Can you work these out from the model? Positions are in its coordinate system, mm. A direction names the side the tool comes from. Give positions to 0.01 mm unless a question says otherwise; leave off trailing zeros. Order: outer loops, then holes, each group sorted by start corner. A loop starts at its lowest first (then second) coordinate and runs counter-clockwise, first axis right, second up. Notation, with made-up numbers: M -5.75,36 L 28.25,36 A8 cw 28.25,40 Z; hole C 26,11.5 d7. An arc over 180 degrees is marked long. One line per question, with ' | ' between items. Start each with the question number.
1) For faces 4 (the flat face through (24, 1, 3.175)), 5 (the flat face through (26.035, 1, -2)), 6 (the flat face through (-26.035, 1, -2)), 7 (the flat face through (-9.525, 8, -5)), which set-ups out of +Z, -Z, +X, -X, +Y, -Y let a thin tool reach every point of the face, with its end or its side?
2) If we section it at C-C, the plane z = 2.25: Please give me the cut outline in (x, y) (3 decimals), plus the area to 3 significant figures.
3) Please list where these lines run through material, in increasing order: line 1 along X through (y, z) = (5.5, -2.25) (3 decimals); line 2 along X through (y, z) = (-2.75, 2.25) (3 decimals); line 3 along X through (y, z) = (-12, -0.75) (3 decimals). Write a range as [from, to].
4) I'm going to push flat-ended pins straight in: pin 1 Ø3 at (y, z) = (-5, 4) entering from -X (3 decimals); pin 2 Ø1.6 at (y, z) = (7.5, -5.5) entering from +X (3 decimals); pin 3 Ø3.5 at (x, z) = (-2.5, -5.5) entering from +Y. Where does each tip first touch, or does it pass through?
5) If we section it at B-B, the plane y = -6.75: Please give me the cut outline in (x, z) (3 decimals).
6) If we section it at D-D, the plane x = 20.5: Please give me the cut outline in (y, z), plus the area to 3 significant figures.
7) Thinking about a two-plate mould opening in X: for faces 1 (the flat face through (-21.59, 0, 2)), 2 (the cylindrical face through (-35.43, -12.09, -6.06)), 3 (the flat face through (0, -2, -6.782)), which applies, +X half, -X half, draft (parallel to the pull), parting line (faces both ways), or undercut?
8) If we section it at A-A, the plane x = -31.75: Please give me the cut outline in (y, z).
```python
from build123d import *

# Parameters (mm, degrees)
BOSS_EXTRUDE1_DEPTH = 10.16
SKETCH3_W           = 19.05
SKETCH3_H           = 6.35
CUT_EXTRUDE1_DEPTH  = 19.05
SKETCH4_W           = 72.39
SKETCH4_H           = 12.7
BOSS_EXTRUDE2_DEPTH = 3.81
SKETCH5_R           = 1.5875
CUT_EXTRUDE2_DEPTH  = 43.059163523
FILLET1_R           = 2.54
FILLET2_R           = 0.508
FILLET3_R           = 2.54
FILLET4_R           = 2.54


with BuildPart() as part:
    # Sketch2 → Boss-Extrude1 (new, symmetric)
    with BuildSketch(Plane(origin=(0, 0, 0), x_dir=(1, 0, 0), z_dir=(0, 1, 0))):
        Polygon((22.86, 3.6068), (-22.86, 3.6068), (-22.86, 0), (-21.59, 0), (-21.59, -3.175), (-26.035, -3.175), (-26.035, 6.7818), (26.035, 6.7818), (26.035, -3.175), (21.59, -3.175), (21.59, 0), (22.86, 0), align=None)
    extrude(amount=BOSS_EXTRUDE1_DEPTH, both=True)

    # Sketch3 → Cut-Extrude1 (cut)
    with BuildSketch(Plane.XY.offset(-3.6068)):
        with Locations((0, 6.985)):
            Rectangle(SKETCH3_W, SKETCH3_H)
    extrude(amount=-CUT_EXTRUDE1_DEPTH, mode=Mode.SUBTRACT)

    # Sketch4 → Boss-Extrude2 (add)
    with BuildSketch(Plane.XZ.offset(10.16)):
        with Locations((0, -0.4318)):
            Rectangle(SKETCH4_W, SKETCH4_H)
    extrude(amount=BOSS_EXTRUDE2_DEPTH)

    # Sketch5 → Cut-Extrude2 (cut, through all)
    with BuildSketch(Plane(origin=(0, -10.16, 0), x_dir=(1, 0, 0), z_dir=(0, 1, 0))):
        with Locations(Location((-31.75, 0.4318, 0), (0, 0, 270))):
            Circle(SKETCH5_R)
        with Locations(Location((31.75, 0.4318, 0), (0, 0, 90))):
            Circle(SKETCH5_R)
    extrude(amount=-CUT_EXTRUDE2_DEPTH, mode=Mode.SUBTRACT)

    # Fillet1
    fillet1_edges = [part.edges().sort_by_distance(p)[0] for p in [
        (-23.8125, -10.16, 3.175),
        (-26.035, -10.16, -1.8034),
        (26.035, -10.16, -1.8034),
        (23.8125, -10.16, 3.175),
    ]]
    fillet(fillet1_edges, radius=FILLET1_R)

    # Fillet2
    fillet2_edges = [part.edges().sort_by_distance(p)[0] for p in [
        (0, -10.16, -3.6068),
        (-22.86, -10.16, -1.8034),
        (-22.86, 0, 0),
        (22.86, 0, 0),
        (22.86, 0, -3.6068),
        (-22.86, 0, -3.6068),
    ]]
    fillet(fillet2_edges, radius=FILLET2_R)

    # Fillet3
    fillet3_edges = [part.edges().sort_by_distance(p)[0] for p in [
        (9.525, 3.81, -5.1943),
        (-9.525, 3.81, -5.1943),
    ]]
    fillet(fillet3_edges, radius=FILLET3_R)

    # Fillet4
    fillet4_edges = [part.edges().sort_by_distance(p)[0] for p in [
        (-36.195, -12.065, 5.9182),
        (-36.195, -12.065, -6.7818),
        (36.195, -12.065, -6.7818),
        (36.195, -12.065, 5.9182),
    ]]
    fillet(fillet4_edges, radius=FILLET4_R)


solid = part.part
```
Results found:
1) face 4: +Z, +X, -X, +Y | face 5: +Z, -Z, +X, +Y | face 6: +Z, -Z, -X, +Y | face 7: +Z, -Z, +Y
2) outline: M -36.195,-13.97 L 36.195,-13.97 L 36.195,-10.16 L 28.575,-10.16 A2.54 cw 26.035,-7.62 L 26.035,10.16 L 21.59,10.16 L 21.59,-10.16 L -21.59,-10.16 L -21.59,10.16 L -26.035,10.16 L -26.035,-7.62 A2.54 cw -28.575,-10.16 L -36.195,-10.16 Z | area: 459 mm²
3) line 1: x = [-26.035, -22.86], [22.86, 26.035] | line 2: x = [-26.035, -21.59], [21.59, 26.035] | line 3: x = [-36.195, -33.305], [-30.195, 30.195], [33.305, 36.195]
4) pin 1: stops at x = -26.035 | pin 2: stops at x = 26.035 | pin 3: stops at y = 3.81
5) outline: M -26.035,-6.782 L 26.035,-6.782 L 26.035,3.175 L 21.59,3.175 L 21.59,0 L 22.352,0 A0.508 cw 22.86,-0.508 L 22.86,-3.099 A0.508 cw 22.352,-3.607 L -22.352,-3.607 A0.508 cw -22.86,-3.099 L -22.86,-0.508 A0.508 cw -22.352,0 L -21.59,0 L -21.59,3.175 L -26.035,3.175 Z
6) outline: M -13.97,-6.78 L 10.16,-6.78 L 10.16,-3.61 L -9.65,-3.61 A0.51 cw -10.16,-3.1 L -10.16,5.92 L -13.97,5.92 Z | area: 113 mm²
7) face 1: undercut | face 2: -X half | face 3: draft
8) outline: M -13.97,-6.78 L -10.16,-6.78 L -10.16,-2.02 L -13.97,-2.02 Z; M -13.97,1.16 L -10.16,1.16 L -10.16,5.92 L -13.97,5.92 Z
